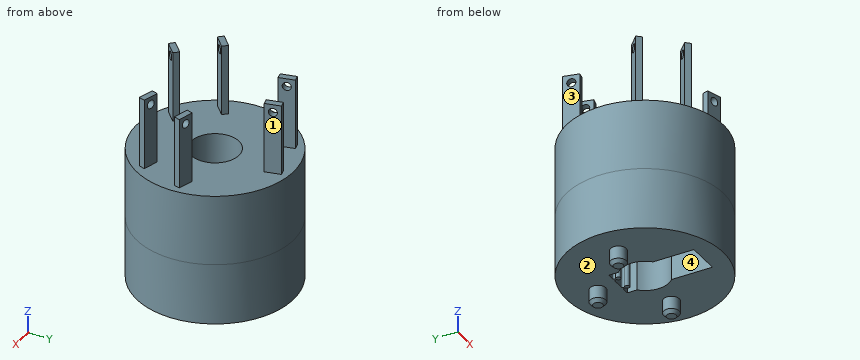
```python
from build123d import *
from build123d.topology import SkipClean

# Parameters (mm, degrees)
SKETCH1_R               = 50
SKETCH3_R               = 50
BOSS_EXTRUDE1_DEPTH     = 45
SKETCH21_R              = 15.25
CUT_EXTRUDE1_DEPTH      = 115.45523151
CUT_EXTRUDE1_DEPTH_BACK = 115.45523151
SKETCH23_W              = 2.65
SKETCH23_H              = 49.393967623
M5_CLEARANCE_HOLE8_D    = 5.3
SKETCH27_W              = 2.65
SKETCH27_H              = 60.041961507
M5_CLEARANCE_HOLE10_D   = 5.3
SKETCH32_W              = 2.65
SKETCH32_H              = 51.511335507
M5_CLEARANCE_HOLE12_D   = 5.3
SKETCH35_R              = 50
BOSS_EXTRUDE2_DEPTH     = 39
SKETCH36_R              = 5
BOSS_EXTRUDE3_DEPTH     = 10
CHAMFER1_SIZE           = 2


with BuildPart() as part:
    # Sketch1 → Loft1 section 0
    with BuildSketch(Plane.XY):
        Circle(SKETCH1_R)
    # Sketch3 → Loft1 section 1
    with BuildSketch(Plane.XY.offset(45)):
        Circle(SKETCH3_R)
    loft()

    # Sketch4 → Boss-Extrude1 (add)
    with BuildSketch(Plane.XY.offset(45)):
        Polygon((-21.649255971, 39.042410979), (-25.54010328, 38.114344591), (-23.21993731, 28.387226319), (-19.329090001, 29.315292707), align=None)
        Polygon((1.695827881, 44.610809306), (5.58667519, 45.538875693), (7.90684116, 35.811757422), (4.015993851, 34.883691034), align=None)
        Polygon((35.016664181, 1.962066431), (36.158358767, 5.795672237), (45.74237328, 2.941435772), (44.600678694, -0.892170034), align=None)
        Polygon((28.166496664, -21.039568402), (27.024802078, -24.873174207), (36.608816592, -27.727410673), (37.750511178, -23.893804867), align=None)
        Polygon((-22.987090484, -38.270012468), (-20.237937762, -41.175551885), (-12.974089217, -34.302670079), (-15.72324194, -31.397130661), align=None)
        Polygon((-39.48200682, -20.836775962), (-42.231159542, -17.931236544), (-34.967310998, -11.058354737), (-32.218158276, -13.963894155), align=None)
    extrude(amount=BOSS_EXTRUDE1_DEPTH)

    # Sketch21 → Cut-Extrude1 (cut, two sides)
    with BuildSketch(Plane(origin=(0, 0, 0), x_dir=(-1, 0, 0), z_dir=(0, 0, -1))) as cut_extrude1_sk:
        Circle(SKETCH21_R)
    extrude(amount=CUT_EXTRUDE1_DEPTH, mode=Mode.SUBTRACT)
    extrude(cut_extrude1_sk.sketch, amount=-CUT_EXTRUDE1_DEPTH_BACK, mode=Mode.SUBTRACT)

    # Sketch23 → M5 Clearance Hole7 (revolve, cut)
    with BuildSketch(Plane(origin=(2.855910866, 39.74725017, 85), x_dir=(0.23201659695614316, -0.9727118271805328, 0), z_dir=(0, 0, 1))):
        with Locations((1.325, 24.696983812)):
            Rectangle(SKETCH23_W, SKETCH23_H)
    revolve(axis=Axis((-3.320809236, 38.273944779, 85), (0.9727118271805328, 0.23201659695614313, 0)), mode=Mode.SUBTRACT)

    # M5 Clearance Hole8 (through all)
    with Locations(Plane(origin=(-11.672541926, -2.784199164, 0), x_dir=(0, 0, -1), z_dir=(0.9727118271805437, 0.23201659695609775, 0))):
        with Locations((-85, 38.000001617)):
            Hole(M5_CLEARANCE_HOLE8_D / 2)

    # Sketch27 → M5 Clearance Hole9 (revolve, cut)
    with BuildSketch(Plane(origin=(-35.850082548, -17.400335058, 85), x_dir=(0.7263848544218454, 0.687288180653905, 0), z_dir=(0, 0, 1))):
        with Locations((1.325, 30.020980754)):
            Rectangle(SKETCH27_W, SKETCH27_H)
    revolve(axis=Axis((-31.485802601, -22.012878884, 85), (-0.6872881806539048, 0.7263848544218454, 0)), mode=Mode.SUBTRACT)

    # M5 Clearance Hole10 (through all)
    with Locations(Plane(origin=(8.247459431, -8.716619588, 0), x_dir=(0.726384854421872, 0.6872881806538769, 0), z_dir=(-0.6872881806538769, 0.726384854421872, 0))):
        with Locations((-38.000001617, -85)):
            Hole(M5_CLEARANCE_HOLE10_D / 2)

    # Sketch32 → M5 Clearance Hole11 (revolve, cut)
    with BuildSketch(Plane(origin=(39.808671437, 0.534948199, 85), x_dir=(0.9584014513779905, -0.28542364652663516, 0), z_dir=(0, 0, 1))):
        with Locations((1.325, 25.755667754)):
            Rectangle(SKETCH32_W, SKETCH32_H)
    revolve(axis=Axis((37.996231282, -5.550901018, 85), (0.2854236465266351, 0.9584014513779905, 0)), mode=Mode.SUBTRACT)

    # M5 Clearance Hole12 (through all)
    with Locations(Plane(origin=(-3.460752782, -11.620587605, 0), x_dir=(0.9584014513779878, -0.28542364652664387, 0), z_dir=(0.28542364652664387, 0.9584014513779878, 0))):
        with Locations((38.000001617, -85)):
            Hole(M5_CLEARANCE_HOLE12_D / 2)

    # Sketch35 → Boss-Extrude2 (add)
    with SkipClean():  # the faces are left unmerged after this step: merging them gives an invalid solid
        with BuildSketch(Plane(origin=(0, 0, 0), x_dir=(-1, 0, 0), z_dir=(0, 0, -1))):
            with Locations(Location((0, 0, 0), (0, 0, 180))):
                Circle(SKETCH35_R)
            with BuildLine():
                ThreePointArc((-4.1, 15.35), (-4.448683298, 16.466227766), (-3.5, 17.15))
                Line((-3.5, 17.15), (3.5, 17.15))
                ThreePointArc((3.5, 17.15), (4.448683298, 16.466227766), (4.1, 15.35))
                ThreePointArc((4.1, 15.35), (5, 12.65), (5.9, 15.35))
                ThreePointArc((5.9, 15.35), (5.551316702, 16.466227766), (6.5, 17.15))
                Line((6.5, 17.15), (10.5, 17.15))
                Line((10.5, 17.15), (10.5, 11.05949818))
                ThreePointArc((10.5, 11.05949818), (15.25, 0), (10.5, -11.05949818))
                Line((10.5, -11.05949818), (10.5, -37.15))
                Line((10.5, -37.15), (-10.5, -37.15))
                Line((-10.5, -37.15), (-10.5, -11.05949818))
                ThreePointArc((-10.5, -11.05949818), (-15.25, 0), (-10.5, 11.05949818))
                Line((-10.5, 11.05949818), (-10.5, 17.15))
                Line((-10.5, 17.15), (-6.5, 17.15))
                ThreePointArc((-6.5, 17.15), (-5.551316702, 16.466227766), (-5.9, 15.35))
                ThreePointArc((-5.9, 15.35), (-5, 12.65), (-4.1, 15.35))
            make_face(mode=Mode.SUBTRACT)
        extrude(amount=BOSS_EXTRUDE2_DEPTH)

    # Sketch36 → Boss-Extrude3 (add)
    with SkipClean():  # the faces are left unmerged after this step: merging them gives an invalid solid
        with BuildSketch(Plane(origin=(0, 0, -39), x_dir=(-1, 0, 0), z_dir=(0, 0, -1))):
            with Locations((0, 30)):
                Circle(SKETCH36_R)
            with Locations((-30, 0)):
                Circle(SKETCH36_R)
            with Locations((30, 0)):
                Circle(SKETCH36_R)
        extrude(amount=BOSS_EXTRUDE3_DEPTH)

    # Chamfer1
    chamfer1_edges = [part.edges().sort_by_distance(p)[0] for p in [
        (5, 30, -49),
        (35, 0, -49),
        (-25, 0, -49),
    ]]
    chamfer(chamfer1_edges, length=CHAMFER1_SIZE)


solid = part.part
```
Geometry: final body of the model. Coordinates: model frame, mm. Face numbers are marked on the shaded views. Coordinates: 2 decimals unless noted, no trailing zeros. Loops run counter-clockwise (first coordinate to the right, second up) from the corner with the lowest first, then second, coordinate; pieces in that order, holes last. Notation, with made-up numbers: (-29, -13.75) -> (19, -13.75) arc R21 cw to (19, 9.25) -> close; hole circle Ø8 at (-27, 23.25). An arc over 180 degrees is marked (long way). Use a Markdown table: item, result. Add a question column.
(1) Section query C-C, the plane y = 22. Return loops of the section in (x, z).
(2) Section query A-A, the plane z = -11.5. Return loops of the section in (x, y).
(3) Pin query (flat end, axial travel): pin 1 Ø5 at (x, y) = (38.5, 25.5) entering from +Z; pin 2 Ø13 at (y, z) = (-20.5, -11) entering from +X; pin 3 Ø6.5 at (y, z) = (15, -22.5) entering from -X. Return the tip coordinate at first contact, or that it passes through.
(4) Line query: line 1 along Y through (x, z) = (0, 35); line 2 along X through (y, z) = (15, -32.5); line 3 along Z through (x, y) = (14.5, -40). Output: solid intervals per line, ascending.
(5) Mould query, pull axis Y, two halves, no side actions, for the marked faces 1, 2, 3 and 4. Classes: pulls with the +Y half, pulls with the -Y half, needs draft (parallel to the pull), parting line crosses it, or undercut.
(6) Section query B-B, the plane x = -30. Return loops of the section in (y, z).
Answer:
| question | item | result |
|---|---|---|
| 1 | outline | (-44.9, -39) -> (44.9, -39) -> (44.9, 45) -> (-44.9, 45) -> close |
| 2 | outline | circle Ø100 at (0, 0); hole (-10.5, -37.15) -> (10.5, -37.15) -> (10.5, -11.06) arc R15.25 ccw to (10.5, 11.06) -> (10.5, 17.15) -> (6.5, 17.15) arc R1 ccw to (5.9, 15.35) arc R1.5 cw (long way) to (4.1, 15.35) arc R1 ccw to (3.5, 17.15) -> (-3.5, 17.15) arc R1 ccw to (-4.1, 15.35) arc R1.5 cw (long way) to (-5.9, 15.35) arc R1 ccw to (-6.5, 17.15) -> (-10.5, 17.15) -> (-10.5, 11.06) arc R15.25 ccw to (-10.5, -11.06) -> close |
| 3 | pin 1 | stops at z = 45 |
| 3 | pin 2 | stops at x = 48 |
| 3 | pin 3 | stops at x = -48.6 |
| 4 | line 1 | y = -50 to -15.25, 15.25 to 50 |
| 4 | line 2 | x = -47.7 to -10.5, -6.24 to -3.76, 3.76 to 6.24, 10.5 to 47.7 |
| 4 | line 3 | z = -39 to 45 |
| 5 | face 1 | pulls with the +Y half |
| 5 | face 2 | needs draft |
| 5 | face 3 | pulls with the -Y half |
| 5 | face 4 | undercut |
| 6 | outline | (-40, -39) -> (-5, -39) -> (-5, -47) -> (-3, -49) -> (3, -49) -> (5, -47) -> (5, -39) -> (40, -39) -> (40, 45) -> (-40, 45) -> close |
